Here's the drawing with two shaded views (mm, measured from the low corner). I have some questions. Coordinates: 2 decimals unless noted, no trailing zeros. Write each loop counter-clockwise with the first axis right and the second up, starting at its lowest first coordinate (ties: lowest second). Pieces come first, ordered by that corner, then holes.
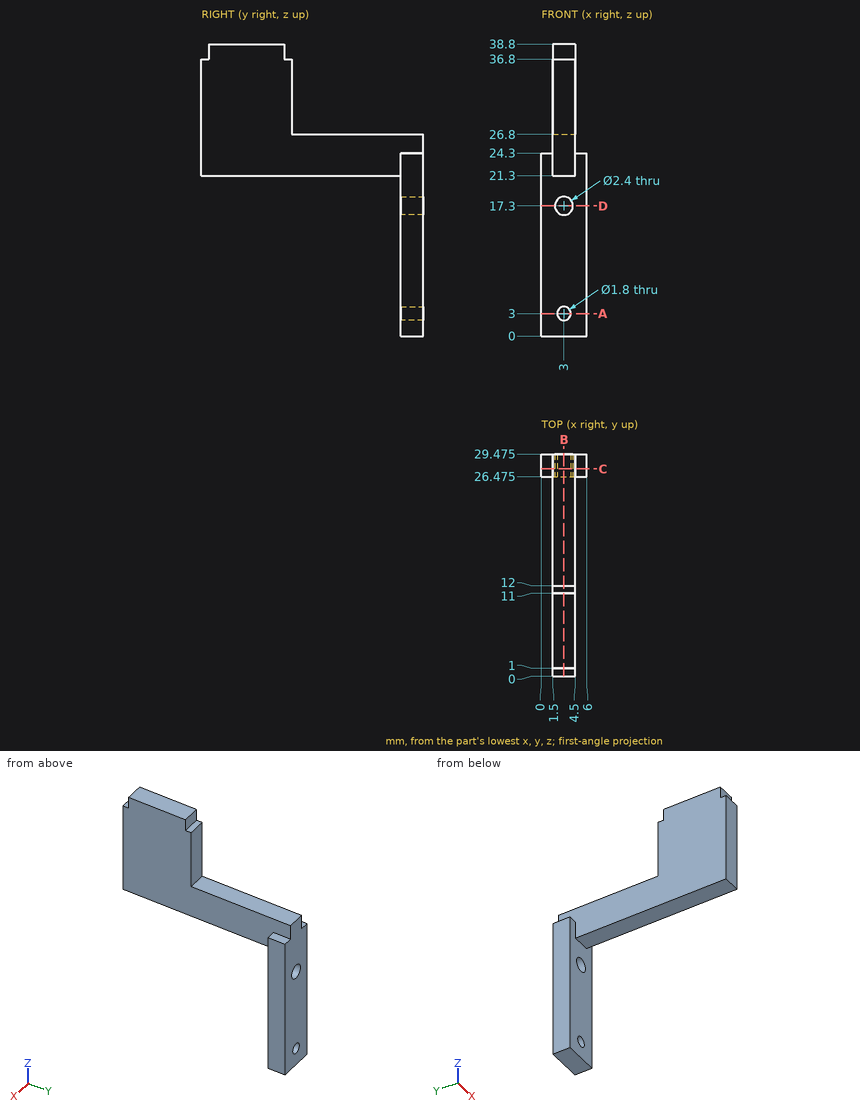
1. I want a section at C-C on y = 27.5. Please give me the cut outline in (x, z).
Verdict:
outline: (0, 0) - (6, 0) - (6, 24.3) - (4.5, 24.3) - (4.5, 26.8) - (1.5, 26.8) - (1.5, 24.3) - (0, 24.3) - close; hole circle Ø2.4 at (3, 17.3); hole circle Ø1.8 at (3, 3)
2. I want a section at D-D on z = 17.3. Please give me the cut outline in (x, y) (3 decimals).
Verdict:
outline: (0, 26.475) - (1.8, 26.475) - (1.8, 29.475) - (0, 29.475) - close; (4.2, 26.475) - (6, 26.475) - (6, 29.475) - (4.2, 29.475) - close
3. Please list where these lines run through material, in increasing order: line 1 along Z through (x, y) = (3, 27.2); line 2 along X through (y, z) = (28, 17.3); line 3 along X through (y, z) = (28.9, 3).
Verdict:
line 1: z = 0 to 2.1, 3.9 to 16.1, 18.5 to 26.8
line 2: x = 0 to 1.8, 4.2 to 6
line 3: x = 0 to 2.1, 3.9 to 6
4. I want a section at B-B on x = 3. Please give me the cut outline in (y, z) (3 decimals).
Verdict:
outline: (0, 21.3) - (26.475, 21.3) - (26.475, 18.5) - (29.475, 18.5) - (29.475, 26.8) - (12, 26.8) - (12, 36.8) - (11, 36.8) - (11, 38.8) - (1, 38.8) - (1, 36.8) - (0, 36.8) - close; (26.475, 0) - (29.475, 0) - (29.475, 2.1) - (26.475, 2.1) - close; (26.475, 3.9) - (29.475, 3.9) - (29.475, 16.1) - (26.475, 16.1) - close
5. I want a section at A-A on z = 3. Please give me the cut outline in (x, y) (3 decimals).
Verdict:
outline: (0, 26.475) - (2.1, 26.475) - (2.1, 29.475) - (0, 29.475) - close; (3.9, 26.475) - (6, 26.475) - (6, 29.475) - (3.9, 29.475) - close
6. For pin 1 (1.6 mm diameter, centred on x = 2.5, z = 37.5, fed in from +Y); pin 2 (14 mm diameter, centred on y = 15.5, z = 28.5, fed in from +X); pin 3 (2.5 mm diameter, centred on x = 3.5, y = 22.5, fed in from +Z), each with a flat end and sliding along its axis, tell me the tip position at first contact or that it passes through.
Verdict:
pin 1: stops at y = 12
pin 2: stops at x = 4.5
pin 3: stops at z = 26.8
